The drawing under review shows one solid part. Ordinate dimensions are in mm from its lowest x, y, z. Give positions to 0.01 mm unless a question says otherwise; leave off trailing zeros. Write each loop counter-clockwise with the first axis right and the second up, starting at its lowest first coordinate (ties: lowest second). Pieces come first, ordered by that corner, then holes. Notation, with made-up numbers: (48, -12) -> (70, -12) arc R27 cw to (70, 19) -> close; hole circle Ø9 at (43, -13.5). An arc over 180 degrees is marked (long way). Answer as a JSON object with one key per item and string values.
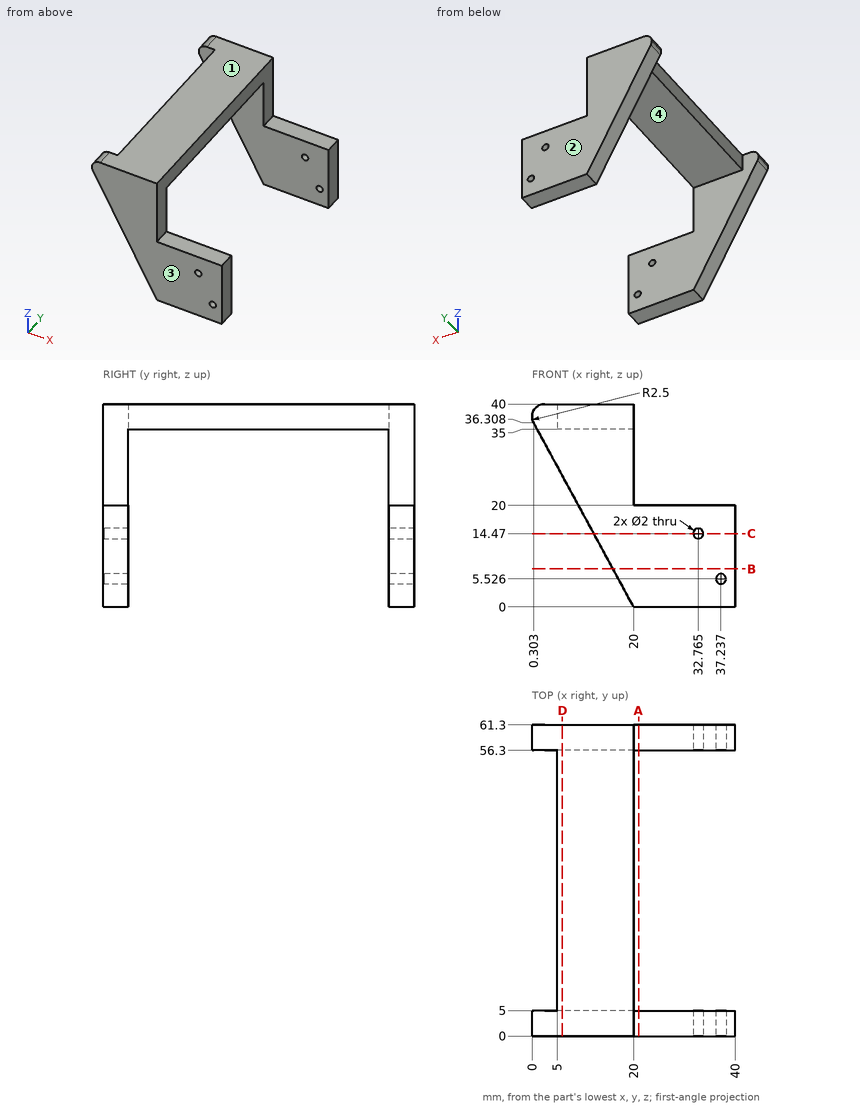
(1) We need section C-C, the plane z = 14.47. Give the number of separate pieces and of enclosed holes in the cut face.
Here are the results:
{"separate pieces": "4", "enclosed holes": "0"}
(2) We need section B-B, the plane z = 7.5. State the section outline as (x, y) points, then the cut area to 3 significant figures.
Here are the results:
{"outline": "(15.93, 0) -> (40, 0) -> (40, 5) -> (15.93, 5) -> close; (15.93, 56.3) -> (40, 56.3) -> (40, 61.3) -> (15.93, 61.3) -> close", "area": "241 mm²"}
(3) Clearance check with flat-ended pins moving along their axes: pin 1 (1 mm diameter, centred on x = 16, y = 36, fed in from -Z); pin 2 (5.5 mm diameter, centred on x = 32, y = 58.5, fed in from +Z); pin 3 (22 mm diameter, centred on y = 31.5, z = 29, fed in from +X). State where each tip first meets the part, or that it passes through.
Here are the results:
{"pin 1": "stops at z = 35", "pin 2": "stops at z = 20", "pin 3": "stops at x = 20"}
(4) The part is to be moulded in two halves that separate along Y. For the marked faces 1, 2, 3 and 4, say which applies: +Y half, -Y half, draft (parallel to the pull), parting line (faces both ways), or undercut.
Here are the results:
{"face 1": "draft", "face 2": "+Y half", "face 3": "-Y half", "face 4": "undercut"}
(5) We need section A-A, the plane x = 21. State the section outline as (y, z) points.
Here are the results:
{"outline": "(0, 0) -> (5, 0) -> (5, 20) -> (0, 20) -> close; (56.3, 0) -> (61.3, 0) -> (61.3, 20) -> (56.3, 20) -> close"}
(6) We need section D-D, the plane x = 6. State the section outline as (y, z) points (1 decimal).
Here are the results:
{"outline": "(0, 25.8) -> (5, 25.8) -> (5, 35) -> (56.3, 35) -> (56.3, 25.8) -> (61.3, 25.8) -> (61.3, 40) -> (0, 40) -> close"}
(7) For line 1 along Y through (x, z) = (15, 31); line 2 along Z through (x, y) = (6, 25.5); line 3 along X through (y, z) = (3, 14) (1 decimal), list the stretches that pass through material, from the lowest coordinate up.
Here are the results:
{"line 1": "y = 0 to 5, 56.3 to 61.3", "line 2": "z = 35 to 40", "line 3": "x = 12.4 to 31.9, 33.6 to 40"}
